Input: part model. Units: mm. Frame: model coordinates. A direction names the side the tool comes from. Round coordinates to 2 decimals unless told otherwise and drop trailing zeros. Loops run counter-clockwise (first coordinate to the right, second up) from the corner with the lowest first, then second, coordinate; pieces in that order, holes last. Notation, with made-up numbers: (-7, -15.5) - (32, -15.5) arc R14 cw to (32, -10.5) - close; hole circle Ø2 at (62.25, 69.5). An arc over 180 degrees is marked (long way). Use CSV: the item, a comma, the result in double quotes. Start each with the question number.
1. Access query for faces 5 (the flat face through (12.35, -16, -61)), 6 (the cylindrical face through (10.89, 105.43, -35.79)), 7 (the flat face through (3, -56.1, -73.5)). Directions: +Z, -Z, +X, -X, +Y, -Y. A direction counts if a zero-diameter tool reaches every point of the face in a straight line with its end or side. Return the directions, or none.
2. Pin query (flat end, axial travel): P1, Ø8, axis at x = 9.5, z = -100, coming from the +Y side; P2, Ø24.5, axis at y = 97.01, z = 40.18, coming from the +X side; P3, Ø1.5, axis at y = -65, z = -76.5, coming from the -X side; P4, Ø2, axis at y = -64.5, z = 47, coming from the -X side. Return the tip coordinate at first contact, or that it passes through.
3. Cut plane A-A (y = 0). Return loops of the section in (x, z).
4. Pull-direction query (Y, two-part tool) for faces 1 (the cylindrical face through (11.11, -124.88, 5.5)), 2 (the cylindrical face through (10.89, -105.43, 35.79)), 3 (the cylindrical face through (10.89, 35.79, 105.43)), 4 (the flat face through (19, 82, -26)); classes: +Y half, -Y half, draft (parallel to the pull), parting line (faces both ways), or undercut.
5. Cut plane D-D (y = 45.5). Return loops of the section in (x, z).
6. Cut plane B-B (z = -41.5). Return loops of the section in (x, y), and give its area (3 significant figures).
7. Material intervals for probe 1 along Y at (x, z) = (6.75, -40); probe 2 along Z at (x, y) = (6.75, 0); probe 3 along Y at (x, z) = (6.5, -96), sorted ascending. Write a range as from..to.
Autodesk Inventor part; units mm, degrees
ref_plane "YZ Plane" through (0, 0, 0) normal (1, 0, 0) x (0, 1, 0)
ref_plane "XZ Plane" through (0, 0, 0) normal (0, 1, 0) x (-1, 0, 0)
ref_plane "XY Plane" through (0, 0, 0) normal (0, 0, 1) x (1, 0, 0)
sketch "Sketch1" plane through (0, 0, 0) normal (0, 0, 1) x (1, 0, 0)
  line L0 (0, 0) -> (24.7, 0) construction
  line L1 (0, 92) -> (3, 92)
  line L2 (3, 125) -> (19, 125)
  line L3 (3, 125) -> (3, 92)
  line L4 (19, 125) -> (19, 85)
  line L5 (24.7, 68.5) -> (24.7, 0) construction
  line L6 (19, 85) -> (24.7, 85)
  line L7 (24.7, 85) -> (24.7, 68.5)
  line L8 (24.7, 68.5) -> (12.35, 68.5)
  line L9 (12.35, 68.5) -> (12.35, 62.5)
  line L10 (12.35, 62.5) -> (0, 62.5)
  line L11 (0, 62.5) -> (0, 0) construction
  line L12 (0, 92) -> (0, 62.5)
  dimension "d0" = 184
  dimension "d1" = 250
  dimension "d2" = 170
  dimension "d7" = 137
  dimension "d8" = 125
  dimension "d9" = 19
  dimension "d10" = 3
  dimension "d12" = 12.35
  dimension "d13" = 24.7
revolve "Revolution1" add sketch "Sketch1" angle 360 about axis through (0, 0, 0) along (1, 0, 0)
sketch "Sketch2" plane through (3, 0, 0) normal (-1, 0, 0) x (0, 0, 1)
  circle A0 centre (0, 0) radius 92
  line L0 (0, 0) -> (0, 105) construction
  circle A1 centre (0, 0) radius 125
  circle A2 centre (0, 0) radius 105 construction
  line L1 (0, 0) -> (40.1818, 97.0074) construction
  circle A3 centre (40.1818, 97.0074) radius 9.5
  dimension "d14" = 19
  dimension "d15" = 105
  dimension "d16" = 22.5
extrude "Extrusion1" cut sketch "Sketch2" against normal blind 19 contours A3
pattern_circular "Circular Pattern1" count 8 over 360 about axis through (1.5, 0, 0) along (1, 0, 0) of "Extrusion1"
equation "\"d0\" = D1"
equation "\"d1\" = D"
equation "\"d2\" = N3"
equation "\"d7\" = ID + 2 * t"
equation "\"d8\" = ID"
equation "\"d9\" = C1"
equation "\"d10\" = F1"
equation "\"d12\" = 0.65 * C1"
equation "\"d13\" = 1.3 * C1"
equation "\"d14\" = L"
equation "\"d15\" = 0.5 * K1"
equation "\"d3\" = C1"
equation "\"C1\" = 19"
equation "\"D\" = 250"
equation "\"L\" = 19"
equation "\"N3\" = 170"
equation "\"D1\" = 184"
equation "\"H1\" = 17"
equation "\"F1\" = 3"
equation "\"ID\" = 125"
equation "\"t\" = 6"
equation "\"Size_Designation\" = 1.2345"
properties part number "DIN EN 1092-2 Hubbed Socket Welding Flange Type 14 - PN 16 Ductile Iron DN125" material "Iron, Ductile"
Established:
1,face 5,"+X"
1,face 6,"+X, -X"
1,face 7,"-X"
2,P1,"stops at y = 80.06"
2,P2,"stops at x = 19"
2,P3,"stops at x = 3"
2,P4,"stops at x = 0"
3,outline,"(0, -92) - (3, -92) - (3, -125) - (19, -125) - (19, -85) - (24.7, -85) - (24.7, -68.5) - (12.35, -68.5) - (12.35, -62.5) - (0, -62.5) - close; (0, 62.5) - (12.35, 62.5) - (12.35, 68.5) - (24.7, 68.5) - (24.7, 85) - (19, 85) - (19, 125) - (3, 125) - (3, 92) - (0, 92) - close"
4,face 1,"parting line"
4,face 2,"undercut"
4,face 3,"undercut"
4,face 4,"draft"
5,outline,"(0, -79.96) - (3, -79.96) - (3, -89.14) - (19, -89.14) - (19, -71.8) - (24.7, -71.8) - (24.7, -51.21) - (12.35, -51.21) - (12.35, -42.85) - (0, -42.85) - close; (0, 42.85) - (12.35, 42.85) - (12.35, 51.21) - (24.7, 51.21) - (24.7, 71.8) - (19, 71.8) - (19, 89.14) - (3, 89.14) - (3, 79.96) - (0, 79.96) - close; (3, -116.42) - (19, -116.42) - (19, -104.88) - (3, -104.88) - close; (3, 104.88) - (19, 104.88) - (19, 116.42) - (3, 116.42) - close"
6,outline,"(0, -82.11) - (3, -82.11) - (3, -87.6) - (19, -87.6) - (19, -74.18) - (24.7, -74.18) - (24.7, -54.5) - (12.35, -54.5) - (12.35, -46.73) - (0, -46.73) - close; (0, 46.73) - (12.35, 46.73) - (12.35, 54.5) - (24.7, 54.5) - (24.7, 74.18) - (19, 74.18) - (19, 87.6) - (3, 87.6) - (3, 82.11) - (0, 82.11) - close; (3, -117.91) - (19, -117.91) - (19, -106.42) - (3, -106.42) - close; (3, 106.42) - (19, 106.42) - (19, 117.91) - (3, 117.91) - close"
6,area,"2,010 mm2"
7,probe 1,"y = -118.43..-106.51, -87.51..-48.02, 48.02..87.51, 106.51..118.43"
7,probe 2,"z = -125..-62.5, 62.5..125"
7,probe 3,"y = -80.06..-49.63, -30.74..30.74, 49.63..80.06"
